```python
from build123d import *

# Parameters (mm, degrees)
F0_W     = 130.175
F0_H     = 67.31
F1_DEPTH = 20.5232
F2_W     = 6.35
F2_H     = 9.779
F3_DEPTH = 3.81
F4_R     = 1.778
F5_DEPTH = 25.4


with BuildPart() as f1:
    # F0 (on Top) → F1 (new body)
    with BuildSketch(Plane.XY):
        with Locations((65.0875, 33.655)):
            Rectangle(F0_W, F0_H)
    extrude(amount=F1_DEPTH)

    # F2 (on face) → F3 (join)
    with BuildSketch(Plane.XZ):
        with Locations((124.206, 8.5471)):
            Rectangle(F2_W, F2_H)
    extrude(amount=F3_DEPTH)

    # F4 (on face) → F5 (join)
    with BuildSketch(Plane(origin=(0, 67.31, 0), x_dir=(-1, 0, 0), z_dir=(0, 1, 0))):
        with Locations((-128.3716, 8.4582)):
            Circle(F4_R)
        with Locations((-128.3716, 12.0396)):
            Circle(F4_R)
    extrude(amount=F5_DEPTH)


solid = f1.part
```
Part model, mm, in its own coordinate system. A direction names the side the tool comes from. Round coordinates to 2 decimals unless told otherwise and drop trailing zeros. Loops run counter-clockwise (first coordinate to the right, second up) from the corner with the lowest first, then second, coordinate; pieces in that order, holes last.
1. Slice it at C-C (y = 79). Give the cut face in (x, z), and give its area (3 significant figures).
Solutions:
outline: circle Ø3.56 at (128.37, 8.46); circle Ø3.56 at (128.37, 12.04)
area: 19.9 mm2
2. 3-axis set-ups, long thin cutter, end or side, ignore diameter. For faces 1 (the face through (121.031, -2, 8)), 2 (the face through (130.175, 33, 10)), 3 (the face through (127.381, -2, 8)): which of +Z, -Z, +X, -X, +Y, -Y reach the whole face in a straight line?
Solutions:
face 1: +Z, -Z, -X, -Y
face 2: +Z, -Z, +X, +Y, -Y
face 3: +Z, -Z, +X, -Y
3. Flat gauge pins, fed straight in: pin 1 (10 mm diameter, centred on x = 82, y = 20, fed in from -Z); pin 2 (5 mm diameter, centred on x = 92.5, z = 3.5, fed in from -Y); pin 3 (12 mm diameter, centred on x = 83, z = 12.5, fed in from +Y); pin 4 (1.9 mm diameter, centred on x = 125, y = -2.5, fed in from -Z). Where does each tip first touch, or does it go through?
Solutions:
pin 1: stops at z = 0
pin 2: stops at y = 0
pin 3: stops at y = 67.31
pin 4: stops at z = 3.66
4. Slice it at A-A (z = 5). Give the cut face in (x, y) (3 decimals).
Solutions:
outline: (0, 0) - (121.031, 0) - (121.031, -3.81) - (127.381, -3.81) - (127.381, 0) - (130.175, 0) - (130.175, 67.31) - (0, 67.31) - close
5. Slice it at B-B (x = 52). Give the cut face in (y, z).
Solutions:
outline: (0, 0) - (67.31, 0) - (67.31, 20.52) - (0, 20.52) - close
6. Drill centre line: line 1 along Y through (x, z) = (100, 9). Where is it in solid material? Low to high.
Solutions:
line 1: y = 0 to 67.31
7. Two-plate mould, pull along Z, no slides. Class faces 4 (the face through (129.68, 79.83, 9.66)), 5 (the face through (128, 92.71, 12)), 6 (the face through (124, -2, 3.658)), 7 (the face through (124, -2, 13.437)): pulls with the +Z half, pulls with the -Z half, needs draft (parallel to the pull), parting line crosses it, or undercut.
Solutions:
face 4: undercut
face 5: needs draft
face 6: pulls with the -Z half
face 7: pulls with the +Z half
